Here's how the part is built. I have some questions about the finished solid (model axes, mm). A direction names the side the tool comes from. Round coordinates to 2 decimals unless told otherwise and drop trailing zeros. Write each loop counter-clockwise with the first axis right and the second up, starting at its lowest first coordinate (ties: lowest second). Pieces come first, ordered by that corner, then holes. Notation, with made-up numbers: (57, 28) - (106, 28) arc R16 cw to (106, 42) - close; hole circle Ø9 at (4.25, -39). An arc over 180 degrees is marked (long way). One line per item, written item: value. Start each with the question number.
Item 1: Thinking about a two-plate mould opening in Z: for faces 1 (the face through (-45.606, 12.325, -0.5)), 2 (the face through (5.55, 0.99, -16.28)), 3 (the face through (-26.429, 0.986, -47.407)), 4 (the face through (-36.864, 12, -31)), which applies, released by +Z, released by -Z, zero draft, split by the parting line, or undercut?
Item 2: For faces 5 (the face through (-20, 2, -21)), 6 (the face through (-9, 1, -9.242)), 7 (the face through (-26.16, 12.32, 1.46)), 8 (the face through (-21, 0, -21)), 9 (the face through (-17.39, 12.32, 6.64)), which set-ups out of +Z, -Z, +X, -X, +Y, -Y let a thin tool reach every point of the face, with its end or its side?
Item 3: If I drill on line 1 (X direction, y = 4, z = -31); line 2 (Y direction, x = -27, z = -27); line 3 (X direction, y = 10.5, z = 2), over which ranges is the centre line in solid material (lowest first)?
Item 4: Imagine slicing it at D-D, the plane x = -14. Please give me the cut outline in (y, z), then the cut area to 3 significant figures.
Item 5: Imagine slicing it at B-B, the plane z = -40.5. Please give me the cut outline in (x, y).
Item 6: Imagine slicing it at C-C, the plane y = 17.5. Please give me the cut outline in (x, z).
Item 7: For P1, Ø1, axis at y = 20, z = -36, coming from the +X side; P2, Ø8, axis at y = 14, z = -32, coming from the -X side; P3, Ø8, axis at y = 14, z = -9.5, coming from the -X side; P4, Ø1.7, axis at x = -26.11, z = -14.99, coming from the +Y side, each with a flat end and sliding along its axis, tell me the tip position at first contact or that it passes through.
Item 8: Imagine slicing it at A-A, the plane x = -4. Please give me the cut outline in (y, z).
```python
from build123d import *

# Parameters (mm, degrees)
F0_W     = 5
F0_H     = 42.5
F1_DEPTH = 25
F0_R     = 1.45
F0_R_2   = 13
F2_DEPTH = 2
F3_R     = 2
F4_DEPTH = 25


# Not quite as in the source:
# - a feature names something its author has since deleted; it is built from what else it names


with BuildPart() as f1:
    # F0 (on Front) → F1 (new body)
    with BuildSketch(Plane.XZ):
        Polygon((-51.006380532, 4.9005637974), (-36.8642449083, -9.2415718264), (-31.8642449083, -9.2415718264), (-29.7931770964, -9.2415718264), (-33.3287110023, -5.7060379204), (-47.4708466261, 8.4360977033), align=None)
        with Locations((-34.3642449083, -30.4915718264)):
            Rectangle(F0_W, F0_H)
        Polygon((-33.3287110023, -5.7060379204), (-29.7931770964, -9.2415718264), (-15.6510414727, 4.9005637974), (-19.1865753786, 8.4360977033), align=None)
    extrude(amount=-F1_DEPTH)

    # F0 (on Front) → F2 (join)
    with BuildSketch(Plane.XZ):
        Polygon((-29.7931770964, -9.2415718264), (-31.8642449083, -9.2415718264), (-31.8642449083, -51.7415718264), (10.6357550917, -51.7415718264), (10.6357550917, -9.2415718264), align=None)
        with Locations((-26.1142449083, -45.9915718264)):
            Circle(F0_R, mode=Mode.SUBTRACT)
        with Locations((4.8857550917, -45.9915718264)):
            Circle(F0_R, mode=Mode.SUBTRACT)
        with Locations((-10.6142449083, -30.4915718264)):
            Circle(F0_R_2, mode=Mode.SUBTRACT)
        with Locations((-26.1142449083, -14.9915718264)):
            Circle(F0_R, mode=Mode.SUBTRACT)
        with Locations((4.8857550917, -14.9915718264)):
            Circle(F0_R, mode=Mode.SUBTRACT)
    extrude(amount=-F2_DEPTH)

    # F3 (on face) → F4 (cut)
    with BuildSketch(Plane(origin=(-19.5173744614, 0, -19.5173744614), x_dir=(0.7071067812, 0, -0.7071067812), z_dir=(0.7071067812, 0, 0.7071067812))):
        with Locations((-29.5321794507, 12.5)):
            Circle(F3_R)
    extrude(amount=-F4_DEPTH, mode=Mode.SUBTRACT)


solid = f1.part
```
Values follow:
1. face 1: released by -Z
1. face 2: undercut
1. face 3: undercut
1. face 4: zero draft
2. face 5: -Z, +X, +Y
2. face 6: +X, +Y, -Y
2. face 7: +Z, +Y, -Y
2. face 8: +Z, -Z, +X, -X, -Y
2. face 9: +Z, +X, +Y, -Y
3. line 1: x = -36.86 to -31.86
3. line 2: y = 0 to 2
3. line 3: x = -48.11 to -41.03, -25.62 to -18.55
4. outline: (0, -51.74) - (2, -51.74) - (2, -43.04) - (0, -43.04) - close; (0, -17.94) - (2, -17.94) - (2, -9.24) - (0, -9.24) - close
4. area: 34.8 mm^2
5. outline: (-36.86, 0) - (-18.91, 0) - (-18.91, 2) - (-31.86, 2) - (-31.86, 25) - (-36.86, 25) - close; (-2.32, 0) - (10.64, 0) - (10.64, 2) - (-2.32, 2) - close
6. outline: (-51.01, 4.9) - (-36.86, -9.24) - (-36.86, -51.74) - (-31.86, -51.74) - (-31.86, -9.24) - (-29.79, -9.24) - (-15.65, 4.9) - (-19.19, 8.44) - (-33.33, -5.71) - (-47.47, 8.44) - close
7. P1: stops at x = -31.86
7. P2: stops at x = -36.86
7. P3: stops at x = -40.61
7. P4: passes through
8. outline: (0, -51.74) - (2, -51.74) - (2, -41.68) - (0, -41.68) - close; (0, -19.3) - (2, -19.3) - (2, -9.24) - (0, -9.24) - close
